from build123d import *

# Parameters (mm, degrees)
F1_DEPTH     = 1
F2_W         = 61
F2_H         = 110
F3_DEPTH     = 2
F5_DEPTH     = 18
F6_T         = 2
F6_T3_DEPTH  = 114
F6_T5_DEPTH  = 65
F6_T7_DEPTH  = 51
F6_T9_DEPTH  = 93
F6_T12_ANGLE = 90.000000001
F6_T14_ANGLE = 90.000000001
F6_T16_ANGLE = 90.000000001
F6_T18_ANGLE = 90.000000001
F7_R         = 7.25
F8_DEPTH     = 24


# Not quite as in the source:
# - a shell that OpenCascade refuses in one call is made with other operations: the cavity is built on its own and cut out


with BuildPart() as f1:
    # F0 (on Top) → F1 (new body)
    with BuildSketch(Plane.XY):
        with BuildLine():
            ThreePointArc((32.5, 53), (31.3284271247, 55.8284271247), (28.5, 57))
            Line((28.5, 57), (-28.5, 57))
            ThreePointArc((-28.5, 57), (-31.3284271247, 55.8284271247), (-32.5, 53))
            Line((-32.5, 53), (-32.5, -53))
            ThreePointArc((-32.5, -53), (-31.3284271247, -55.8284271247), (-28.5, -57))
            Line((-28.5, -57), (28.5, -57))
            ThreePointArc((28.5, -57), (31.3284271247, -55.8284271247), (32.5, -53))
            Line((32.5, -53), (32.5, 53))
        make_face()
    extrude(amount=F1_DEPTH)

    # F2 (on Top) → F3 (join)
    with BuildSketch(Plane.XY):
        Rectangle(F2_W, F2_H)
    extrude(amount=-F3_DEPTH)

    # F4 (on face) → F5 (join)
    with BuildSketch(Plane(origin=(0, 0, -2), x_dir=(1, 0, 0), z_dir=(0, 0, -1))):
        with BuildLine():
            Line((23.5, 52), (-23.5, 52))
            ThreePointArc((-23.5, 52), (-26.3284271247, 50.8284271247), (-27.5, 48))
            Line((-27.5, 48), (-27.5, -41))
            ThreePointArc((-27.5, -41), (-26.3284271247, -43.8284271247), (-23.5, -45))
            Line((-23.5, -45), (23.5, -45))
            ThreePointArc((23.5, -45), (26.3284271247, -43.8284271247), (27.5, -41))
            Line((27.5, -41), (27.5, 48))
            ThreePointArc((27.5, 48), (26.3284271247, 50.8284271247), (23.5, 52))
        make_face()
    extrude(amount=F5_DEPTH)

    # F6: shell of thickness 2, made by hand


with BuildPart() as f6_core1:
    # F6_t2: copy of F1
    add(f1.part)

    # the walls: a layer under each face that stays
    f6_faces = [f6_core1.faces().sort_by_distance(p)[0] for p in [
        (31.3284271247, 55.8284271247, 0.5),
        (32.5, 0, 0.5),
        (0, 57, 0.5),
        (22.34375, -55.5925925926, 0),
        (31.3284271247, -55.8284271247, 0.5),
        (-31.3284271247, 55.8284271247, 0.5),
        (0, -57, 0.5),
        (-32.5, 0, 0.5),
        (-31.3284271247, -55.8284271247, 0.5),
        (30.5, 0, -1),
        (0, 55, -1),
        (-30.5, 0, -1),
        (0, -55, -1),
        (-26.1428571429, 47.1428571429, -2),
        (26.3284271247, 43.8284271247, -11),
        (0, 45, -11),
        (-26.3284271247, 43.8284271247, -11),
        (-27.5, -3.5, -11),
        (-26.3284271247, -50.8284271247, -11),
        (0, -52, -11),
        (26.3284271247, -50.8284271247, -11),
        (27.5, -3.5, -11),
        (0, -3.5, -20),
    ]]
    thicken(f6_faces, amount=-F6_T, mode=Mode.SUBTRACT)

    # F6_s4 → F6_t3 (cut)
    with BuildSketch(Plane.XZ.offset(-57)):
        Polygon((30.52, -0.02), (30.5, 2), (28.5, 2), (28.5, 0), align=None)
        Polygon((-30.52, -0.02), (-30.5, 2), (-28.5, 2), (-28.5, 0), align=None)
    extrude(amount=F6_T3_DEPTH, mode=Mode.SUBTRACT)

    # F6_s6 → F6_t5 (cut)
    with BuildSketch(Plane.YZ.offset(-32.5)):
        Polygon((55.02, -0.02), (55, 2), (53, 2), (53, 0), align=None)
        Polygon((-55.02, -0.02), (-55, 2), (-53, 2), (-53, 0), align=None)
    extrude(amount=F6_T5_DEPTH, mode=Mode.SUBTRACT)

    # F6_s8 → F6_t7 (cut)
    with BuildSketch(Plane.YZ.offset(-25.5)):
        Polygon((45.02, -2.02), (45, 0), (43, 0), (43, -2), align=None)
        Polygon((-52.02, -2.02), (-52, 0), (-50, 0), (-50, -2), align=None)
    extrude(amount=F6_T7_DEPTH, mode=Mode.SUBTRACT)

    # F6_s10 → F6_t9 (cut)
    with BuildSketch(Plane.XZ.offset(-43)):
        Polygon((-27.52, -2.02), (-27.5, 0), (-25.5, 0), (-25.5, -2), align=None)
        Polygon((27.52, -2.02), (27.5, 0), (25.5, 0), (25.5, -2), align=None)
    extrude(amount=F6_T9_DEPTH, mode=Mode.SUBTRACT)

    # F6_s11 → F6_t12 (revolve, cut)
    with BuildSketch(Plane.YZ.offset(23.5)):
        Polygon((45.02, -2.02), (45, 0), (43, 0), (43, -2), align=None)
    revolve(axis=Axis((23.5, 41, -2), (0, 0, -1)), revolution_arc=F6_T12_ANGLE, mode=Mode.SUBTRACT)

    # F6_s13 → F6_t14 (revolve, cut)
    with BuildSketch(Plane.XZ.offset(-41)):
        Polygon((-27.52, -2.02), (-27.5, 0), (-25.5, 0), (-25.5, -2), align=None)
    revolve(axis=Axis((-23.5, 41, -2), (0, 0, -1)), revolution_arc=F6_T14_ANGLE, mode=Mode.SUBTRACT)

    # F6_s15 → F6_t16 (revolve, cut)
    with BuildSketch(Plane.YZ.offset(-23.5)):
        Polygon((-52.02, -2.02), (-52, 0), (-50, 0), (-50, -2), align=None)
    revolve(axis=Axis((-23.5, -48, -2), (0, 0, -1)), revolution_arc=F6_T16_ANGLE, mode=Mode.SUBTRACT)

    # F6_s17 → F6_t18 (revolve, cut)
    with BuildSketch(Plane.XZ.offset(48)):
        Polygon((27.52, -2.02), (27.5, 0), (25.5, 0), (25.5, -2), align=None)
    revolve(axis=Axis((23.5, -48, -2), (0, 0, -1)), revolution_arc=F6_T18_ANGLE, mode=Mode.SUBTRACT)


with BuildPart() as f1_1:
    add(f1.part)

    # what is left inside the walls is the cavity
    f6_cavity = [f6_core1.part.solids().sort_by_distance(p)[0] for p in [
        (0, -17.666667, 0.98),
    ]]
    add(f6_cavity, mode=Mode.SUBTRACT)

    # F7 (on Right) → F8 (join, symmetric)
    with BuildSketch(Plane.YZ):
        with Locations((35.5, -11)):
            Circle(F7_R)
        with Locations((20, -11)):
            Circle(F7_R)
        with Locations((4.5, -11)):
            Circle(F7_R)
        with Locations((-11, -11)):
            Circle(F7_R)
        with Locations((-26.5, -11)):
            Circle(F7_R)
        with Locations((-42, -11)):
            Circle(F7_R)
    extrude(amount=F8_DEPTH, both=True)


solid = f1_1.part
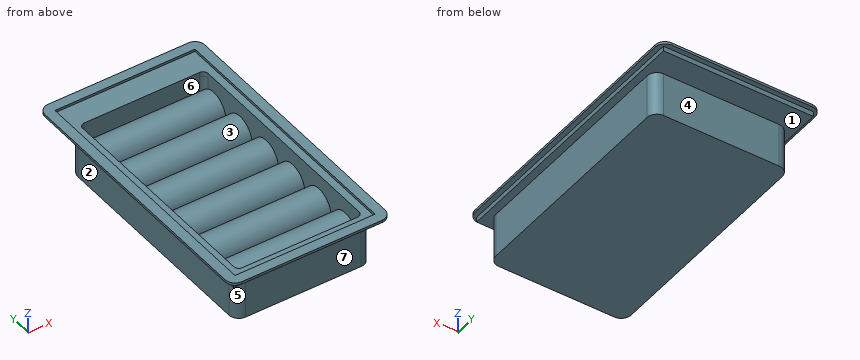
Could you check a few things on this model? Use its own coordinates, in mm. Face numbers are marked on the shaded views. A direction names the side the tool comes from. Give positions to 0.01 mm unless a question says otherwise; leave off trailing zeros. Loops run counter-clockwise (first coordinate to the right, second up) from the corner with the lowest first, then second, coordinate; pieces in that order, holes last. Notation, with made-up numbers: (84, 55.5) -> (143, 55.5) arc R23 cw to (143, 77.5) -> close; hole circle Ø10 at (-29, 17.25). An arc over 180 degrees is marked (long way). Answer as CSV lines item,"result". Start each with the question number.
(1) If we section it at A-A on z = -11: Count the separate pieces of the cut face and the enclosed holes in it, then the cut area to 3 significant figures.
(2) Which directions (+Z, -Z, +X, -X, +Y, -Y) give clear straight access to the entire face, cutting with the end or side of a thin tool? Please do the marked faces 1, 2, 3 and 4.
(3) If we section it at B-B on y = 31: Write out the boundary of the cut face in (x, z), then the cut area to 3 significant figures.
(4) I'm going to push flat-ended pins straight in: pin 1 Ø1 at (x, z) = (-4, -1.5) entering from +Y; pin 2 Ø5 at (x, z) = (-11, -5.5) entering from +Y; pin 3 Ø4.5 at (y, z) = (-10, -12) entering from +X. Where does each tip first touch, or does it pass through?
(5) I need wall thicknesses on probe 1 along X at (y, z) = (-11, -4.75); probe 2 along X at (y, z) = (-19, -11); probe 3 along Z at (x, y) = (29, 46). Which ranges of each line are inside material? Lowest first, please.
(6) We'd pull the mould along X, two halves only. Please class the marked faces 5, 6 and 7: released by +X, released by -X, zero draft, split by the parting line, or undercut.
(7) If we section it at C-C on y = 4.5: Write out the boundary of the cut face in (x, z).
Computed:
1,separate pieces,"7"
1,enclosed holes,"1"
1,area,"4,760 mm2"
2,face 1,"-Z"
2,face 2,"-Z, -X, +Y, -Y"
2,face 3,"none"
2,face 4,"-Z, +X, -X, +Y"
3,outline,"(-32.5, 0) -> (-30.5, 0) -> (-30.5, -2) -> (-27.5, -2) -> (-27.5, -20) -> (27.5, -20) -> (27.5, -2) -> (30.5, -2) -> (30.5, 0) -> (32.5, 0) -> (32.5, 1) -> (28.5, 1) -> (28.5, 0) -> (25.5, 0) -> (25.5, -18) -> (-25.5, -18) -> (-25.5, 0) -> (-28.5, 0) -> (-28.5, 1) -> (-32.5, 1) -> close; (-24, -16.68) -> (24, -16.68) -> (24, -5.32) -> (-24, -5.32) -> close"
3,area,"748 mm2"
4,pin 1,"stops at y = 55"
4,pin 2,"stops at y = 45"
4,pin 3,"stops at x = 27.5"
5,probe 1,"x = -27.5 to -25.5, -24 to 24, 25.5 to 27.5"
5,probe 2,"x = -27.5 to -25.5, 25.5 to 27.5"
5,probe 3,"z = -2 to 1"
6,face 5,"released by -X"
6,face 6,"undercut"
6,face 7,"zero draft"
7,outline,"(-32.5, 0) -> (-30.5, 0) -> (-30.5, -2) -> (-27.5, -2) -> (-27.5, -20) -> (27.5, -20) -> (27.5, -2) -> (30.5, -2) -> (30.5, 0) -> (32.5, 0) -> (32.5, 1) -> (28.5, 1) -> (28.5, 0) -> (25.5, 0) -> (25.5, -18) -> (24, -18) -> (24, -3.75) -> (-24, -3.75) -> (-24, -18) -> (-25.5, -18) -> (-25.5, 0) -> (-28.5, 0) -> (-28.5, 1) -> (-32.5, 1) -> close"
